from build123d import *

# Parameters (mm, degrees)
SKETCH_1_W      = 58
SKETCH_1_H      = 36
SKETCH_1_R      = 1
EXTRUDE_1_DEPTH = 0.8
SKETCH_2_W      = 1.8
SKETCH_2_H      = 1.8
EXTRUDE_2_DEPTH = 1
EXTRUDE_START   = -0.8
SKETCH_2_3_W    = 5.2
SKETCH_2_3_H    = 13
EXTRUDE_3_DEPTH = 5.6
SKETCH_3_W      = 1.5
SKETCH_3_H      = 8.7
EXTRUDE_4_DEPTH = 1
SKETCH_3_3_W    = 7.3
SKETCH_3_3_H    = 14.7
EXTRUDE_5_DEPTH = 10.2
SKETCH_4_W      = 2
SKETCH_4_H      = 2
EXTRUDE_6_DEPTH = 1
SKETCH_4_3_R    = 5.1
EXTRUDE_7_DEPTH = 16.7
SKETCH_5_W      = 3
SKETCH_5_H      = 20
EXTRUDE_8_DEPTH = 1
SKETCH_5_2_W    = 3
SKETCH_5_2_H    = 20
EXTRUDE_9_DEPTH = 1


with BuildPart() as part:
    # 草图1 → 凸台-拉伸1 (new body)
    with BuildSketch(Plane.XY):
        Rectangle(SKETCH_1_W, SKETCH_1_H)
        with Locations((-26, -15)):
            Circle(SKETCH_1_R, mode=Mode.SUBTRACT)
        with Locations((-26, 15)):
            Circle(SKETCH_1_R, mode=Mode.SUBTRACT)
        with Locations((26, 15)):
            Circle(SKETCH_1_R, mode=Mode.SUBTRACT)
        with Locations((26, -15)):
            Circle(SKETCH_1_R, mode=Mode.SUBTRACT)
    extrude(amount=EXTRUDE_1_DEPTH)

    # 草图2 → 凸台-拉伸2 (add)
    with BuildSketch(Plane(origin=(0, 0, 0), x_dir=(-1, 0, 0), z_dir=(0, 0, -1))):
        with Locations((-20.1, -13.1)):
            Rectangle(SKETCH_2_W, SKETCH_2_H)
        with Locations((-20.1, -1.9)):
            Rectangle(SKETCH_2_W, SKETCH_2_H)
        with Locations((-20.1, 1.9)):
            Rectangle(SKETCH_2_W, SKETCH_2_H)
        with Locations((-20.1, 13.1)):
            Rectangle(SKETCH_2_W, SKETCH_2_H)
        with Locations((-14.2, 13.1)):
            Rectangle(SKETCH_2_W, SKETCH_2_H)
        with Locations((-14.2, 1.9)):
            Rectangle(SKETCH_2_W, SKETCH_2_H)
        with Locations((-14.2, -1.9)):
            Rectangle(SKETCH_2_W, SKETCH_2_H)
        with Locations((-14.2, -13.1)):
            Rectangle(SKETCH_2_W, SKETCH_2_H)
    extrude(amount=EXTRUDE_2_DEPTH)

    # 草图2<3> → 凸台-拉伸3 (add)
    with BuildSketch(Plane(origin=(0, 0, 0), x_dir=(-1, 0, 0), z_dir=(0, 0, -1)).offset(EXTRUDE_START)):
        with Locations((-20.1, 7.5)):
            Rectangle(SKETCH_2_3_W, SKETCH_2_3_H)
        with Locations((-14.2, 7.5)):
            Rectangle(SKETCH_2_3_W, SKETCH_2_3_H)
        with Locations((-20.1, -7.5)):
            Rectangle(SKETCH_2_3_W, SKETCH_2_3_H)
        with Locations((-14.2, -7.5)):
            Rectangle(SKETCH_2_3_W, SKETCH_2_3_H)
    extrude(amount=-EXTRUDE_3_DEPTH)

    # 草图3 → 凸台-拉伸4 (add)
    with BuildSketch(Plane(origin=(0, 0, 0), x_dir=(-1, 0, 0), z_dir=(0, 0, -1))):
        with Locations((9.75, 8.85)):
            Rectangle(SKETCH_3_W, SKETCH_3_H)
        with Locations((9.75, -8.85)):
            Rectangle(SKETCH_3_W, SKETCH_3_H)
    extrude(amount=EXTRUDE_4_DEPTH)

    # 草图3<3> → 凸台-拉伸5 (add)
    with BuildSketch(Plane(origin=(0, 0, 0), x_dir=(-1, 0, 0), z_dir=(0, 0, -1)).offset(EXTRUDE_START)):
        with Locations((6.85, 8.85)):
            Rectangle(SKETCH_3_3_W, SKETCH_3_3_H)
        with Locations((6.85, -8.85)):
            Rectangle(SKETCH_3_3_W, SKETCH_3_3_H)
    extrude(amount=-EXTRUDE_5_DEPTH)

    # 草图4 → 凸台-拉伸6 (add)
    with BuildSketch(Plane(origin=(0, 0, 0), x_dir=(-1, 0, 0), z_dir=(0, 0, -1))):
        with Locations((-5.8, 0)):
            Rectangle(SKETCH_4_W, SKETCH_4_H)
        with Locations((-2.8, 0)):
            Rectangle(SKETCH_4_W, SKETCH_4_H)
        with Locations((-5.8, 11.4)):
            Rectangle(SKETCH_4_W, SKETCH_4_H)
        with Locations((-2.8, 11.4)):
            Rectangle(SKETCH_4_W, SKETCH_4_H)
        with Locations((-5.8, -11.4)):
            Rectangle(SKETCH_4_W, SKETCH_4_H)
        with Locations((-2.8, -11.4)):
            Rectangle(SKETCH_4_W, SKETCH_4_H)
    extrude(amount=EXTRUDE_6_DEPTH)

    # 草图4<3> → 凸台-拉伸7 (add)
    with BuildSketch(Plane(origin=(0, 0, 0), x_dir=(-1, 0, 0), z_dir=(0, 0, -1)).offset(EXTRUDE_START)):
        with Locations((-4.3, 0)):
            Circle(SKETCH_4_3_R)
        with Locations((-4.3, 11.4)):
            Circle(SKETCH_4_3_R)
        with Locations((-4.3, -11.4)):
            Circle(SKETCH_4_3_R)
    extrude(amount=-EXTRUDE_7_DEPTH)

    # 草图5 → 凸台-拉伸8 (add)
    with BuildSketch(Plane(origin=(0, 0, 0), x_dir=(-1, 0, 0), z_dir=(0, 0, -1))):
        with Locations((-27.5, 0)):
            Rectangle(SKETCH_5_W, SKETCH_5_H)
    extrude(amount=EXTRUDE_8_DEPTH)

    # 草图5<2> → 凸台-拉伸9 (add)
    with BuildSketch(Plane(origin=(0, 0, 0), x_dir=(-1, 0, 0), z_dir=(0, 0, -1)).offset(EXTRUDE_START)):
        with Locations((-27.5, 0)):
            Rectangle(SKETCH_5_2_W, SKETCH_5_2_H)
    extrude(amount=-EXTRUDE_9_DEPTH)


solid = part.part
Input: part model. Units: mm. Frame: model coordinates. A direction names the side the tool comes from. Give positions to 0.01 mm unless a question says otherwise; leave off trailing zeros. Order: outer loops, then holes, each group sorted by start corner. A loop starts at its lowest first (then second) coordinate and runs counter-clockwise, first axis right, second up.
Q1. Draft query along X for faces 1 (the flat face through (20, 2, -1)), 2 (the flat face through (-3.2, -9, 6)). Return one class per face: +X half, -X half, draft (parallel to the pull), parting line (faces both ways), or undercut.
Checked values:
face 1: draft
face 2: undercut
Q2. Section A-A on x = -26. Output: boundary loops of the cut face in (y, z).
Checked values:
outline: (-18, 0) - (-16, 0) - (-16, 0.8) - (-18, 0.8) - close; (-14, 0) - (14, 0) - (14, 0.8) - (-14, 0.8) - close; (16, 0) - (18, 0) - (18, 0.8) - (16, 0.8) - close
Q3. Ray query, probe 1 along Y at (x, z) = (26, 0.2); probe 2 along Y at (x, z) = (5.5, 4.75); probe 3 along Z at (x, y) = (17, -8.5). Return the intervals inside material, ascending.
Checked values:
probe 1: y = -18 to -16, -14 to 14, 16 to 18
probe 2: y = -16.36 to -6.44, -4.96 to 4.96, 6.44 to 16.36
probe 3: z = 0 to 0.8
Q4. Section B-B on z = 3. State how many separate pieces and enclosed holes the cut face has, and give its area (3 significant figures).
Checked values:
separate pieces: 9
enclosed holes: 0
area: 730 mm2
Q5. Section D-D on z = 11.75. Output: boundary loops of the cut face in (x, y).
Checked values:
outline: circle Ø10.2 at (4.3, -11.4); circle Ø10.2 at (4.3, 0); circle Ø10.2 at (4.3, 11.4)
Q6. Set-up query: faces 3 (the cylindrical face through (1.9, -15.9, 9)), 4 (the flat face through (20, -14, 4)), 5 (the flat face through (17.5, 7, 4)). Return all of +Z, -Z, +X, -X, +Y, -Y with unobstructed straight access to the full face (end or side cutting, diameter ignored); none if empty.
Checked values:
face 3: +Z
face 4: +Z, +X, -Y
face 5: +Z, +Y, -Y
Q7. Contact query for flat-ended pins moving along their axis: pin 1 Ø0.5 at (x, z) = (20, -0.5) entering from +Y; pin 2 Ø11 at (y, z) = (-8.5, 7) entering from +X; pin 3 Ø0.8 at (y, z) = (-2, -0.5) entering from -X; pin 4 Ø1.6 at (x, y) = (26, -15) entering from -Z. Output: stop coordinate, or through.
Checked values:
pin 1: stops at y = 14
pin 2: stops at x = 29
pin 3: stops at x = 13.3
pin 4: passes through
